Source: CAD feature listing. Evaluate the final solid. Frame: model axes, mm. A direction names the side the tool comes from. Coordinates: 2 decimals unless noted, no trailing zeros. Write each loop counter-clockwise with the first axis right and the second up, starting at its lowest first coordinate (ties: lowest second). Pieces come first, ordered by that corner, then holes. Notation, with made-up numbers: (4, -27.5) - (48, -27.5) arc R11 ccw to (48, -17.5) - close; hole circle Ø10 at (29, 27). An arc over 180 degrees is marked (long way). One line per item, written item: value.
from build123d import *

# Parameters (mm, degrees)
SKETCH1_W                 = 6
SKETCH1_H                 = 6
BOSS_EXTRUDE1_DEPTH       = 4
SKETCH2_R                 = 1.6
BOSS_EXTRUDE2_DEPTH       = 1.5
SKETCH3_W                 = 0.7
SKETCH3_H                 = 5
BOSS_EXTRUDE3_DEPTH       = 0.3
LPATTERN2_COUNT           = 2
LPATTERN2_PITCH           = 6.3
LPATTERN3_COUNT           = 2
LPATTERN3_PITCH           = 4.9
LPATTERN3_COPY_1_SKETCH_W = 0.7
LPATTERN3_COPY_1_SKETCH_H = 5
LPATTERN3_COPY_1_DEPTH    = 0.3


with BuildPart() as part:
    # Sketch1 → Boss-Extrude1 (new body)
    with BuildSketch(Plane(origin=(0, 0, 0), x_dir=(1, 0, 0), z_dir=(0, 1, 0))):
        with Locations((3, 3)):
            Rectangle(SKETCH1_W, SKETCH1_H)
    extrude(amount=BOSS_EXTRUDE1_DEPTH)

    # Sketch2 → Boss-Extrude2 (add)
    with BuildSketch(Plane(origin=(0, 4, 0), x_dir=(1, 0, 0), z_dir=(0, 1, 0))):
        with Locations(Location((3, 3, 0), (0, 0, 270))):
            Circle(SKETCH2_R)
    extrude(amount=BOSS_EXTRUDE2_DEPTH)

    # Sketch3 → Boss-Extrude3 (add)
    with BuildSketch(Plane.ZY):
        with Locations((-0.55, -1.5)):
            Rectangle(SKETCH3_W, SKETCH3_H)
    boss_extrude3 = extrude(amount=BOSS_EXTRUDE3_DEPTH)

    # LPattern2: Boss-Extrude3 ×2
    with Locations(*[(i * LPATTERN2_PITCH, 0, 0) for i in range(1, LPATTERN2_COUNT)]):
        add(boss_extrude3)

    # LPattern3: Boss-Extrude3 ×2
    with Locations(*[(0, 0, -i * LPATTERN3_PITCH) for i in range(1, LPATTERN3_COUNT)]):
        add(boss_extrude3)

    # LPattern3 copy 1 sketch → LPattern3 copy 1 (add)
    with BuildSketch(Plane(origin=(6.3, 0, -4.9), x_dir=(0, 0, 1), z_dir=(-1, 0, 0))):
        with Locations((-0.55, -1.5)):
            Rectangle(LPATTERN3_COPY_1_SKETCH_W, LPATTERN3_COPY_1_SKETCH_H)
    extrude(amount=LPATTERN3_COPY_1_DEPTH)


solid = part.part
1) Section query A-A on z = -3. Output: boundary loops of the cut face in (x, y), then the cut area to 3 significant figures.
Values found:
outline: (0, 0) - (6, 0) - (6, 4) - (4.6, 4) - (4.6, 5.5) - (1.4, 5.5) - (1.4, 4) - (0, 4) - close
area: 28.8 mm2
2) Reachability of faces 1 (the flat face through (3, 5.5, -3)), 2 (the flat face through (1.6, 4, -4.4)) from +Z, -Z, +X, -X, +Y, -Y: full face, straight path, thin tool, end or side. Return the list, or none.
Values found:
face 1: +Z, -Z, +X, -X, +Y
face 2: +Y
3) Draft query along Z for faces 3 (the flat face through (3, 0, -3)), 4 (the flat face through (3, 2, -6)), 5 (the flat face through (6, 2, -3)), 6 (the flat face through (3, 2, 0)). Return one class per face: released by +Z, released by -Z, zero draft, split by the parting line, or undercut.
Values found:
face 3: zero draft
face 4: released by -Z
face 5: undercut
face 6: released by +Z
4) Section query D-D on z = -4.9. Output: boundary loops of the cut face in (x, y), then the cut area to 3 significant figures.
Values found:
outline: (0, 0) - (6, 0) - (6, 4) - (0, 4) - close
area: 24.0 mm2
5) Contact query for flat-ended pins moving along their axis: P1, Ø3, axis at x = 4, z = -4, coming from the -Y side; P2, Ø1.5, axis at y = 3, z = -1, coming from the -X side. Output: stop coordinate, or through.
Values found:
P1: y = 0
P2: x = 0
6) Section query B-B on x = 3. Output: boundary loops of the cut face in (y, z).
Values found:
outline: (0, -6) - (4, -6) - (4, -4.6) - (5.5, -4.6) - (5.5, -1.4) - (4, -1.4) - (4, 0) - (0, 0) - close
7) Material intervals for line 1 (Y direction, x = 2, z = -5.65); line 2 (X direction, y = 1.5, z = -5.5); line 3 (Y direction, x = 3, z = -4.15), sorted ascending.
Values found:
line 1: 0 to 4
line 2: 0 to 6
line 3: 0 to 5.5
8) Section query C-C on y = 2.5. Output: boundary loops of the cut face in (x, z), then the cut area to 3 significant figures.
Values found:
outline: (0, -6) - (6, -6) - (6, 0) - (0, 0) - close
area: 36.0 mm2
